Geometry check sheet. Reference: drawing and pictorial views, mm from the part's lowest x, y, z. Coordinates: 2 decimals unless noted, no trailing zeros. Write each loop counter-clockwise with the first axis right and the second up, starting at its lowest first coordinate (ties: lowest second). Pieces come first, ordered by that corner, then holes.
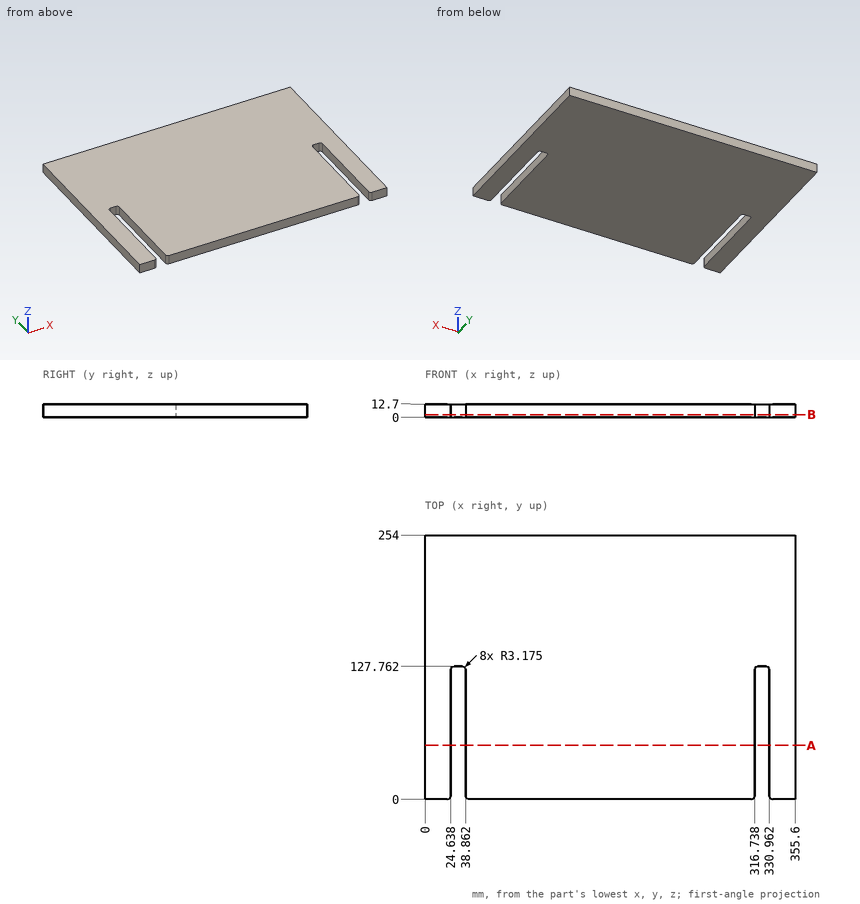
1. Material ranges on L1, parallel to X at y = 24.5, z = 12; L2, parallel to Y at x = 314, z = 0.75; L3, parallel to Y at x = 31, z = 8.5, recorded low to high.
2. Sectioned sample at A-A, the plane y = 52. Record the boundary of the cut face in (x, z).
3. Gauge pin test, flat ends, axial feed: P1, Ø10, axis at x = 106, y = 157.5, coming from the -Z side; P2, Ø6.5, axis at x = 32, z = 8, coming from the -Y side. Record the tip position at first contact, or that the pin passes through.
4. Sectioned sample at B-B, the plane z = 2.5. Record the boundary of the cut face in (x, y) (3 decimals), and give its area (3 significant figures).
Outcome:
1. L1: x = 0 to 24.64, 38.86 to 316.74, 330.96 to 355.6
1. L2: y = 0.03 to 254
1. L3: y = 127.76 to 254
2. outline: (0, 0) - (24.64, 0) - (24.64, 12.7) - (0, 12.7) - close; (38.86, 0) - (316.74, 0) - (316.74, 12.7) - (38.86, 12.7) - close; (330.96, 0) - (355.6, 0) - (355.6, 12.7) - (330.96, 12.7) - close
3. P1: stops at z = 0
3. P2: stops at y = 127.76
4. outline: (0, 0) - (21.463, 0) arc R3.175 ccw to (24.638, 3.175) - (24.638, 124.587) arc R3.175 cw to (27.813, 127.762) - (35.687, 127.762) arc R3.175 cw to (38.862, 124.587) - (38.862, 3.175) arc R3.175 ccw to (42.037, 0) - (313.563, 0) arc R3.175 ccw to (316.738, 3.175) - (316.738, 124.587) arc R3.175 cw to (319.913, 127.762) - (327.787, 127.762) arc R3.175 cw to (330.962, 124.587) - (330.962, 3.175) arc R3.175 ccw to (334.137, 0) - (355.6, 0) - (355.6, 254) - (0, 254) - close
4. area: 86,700 mm2
